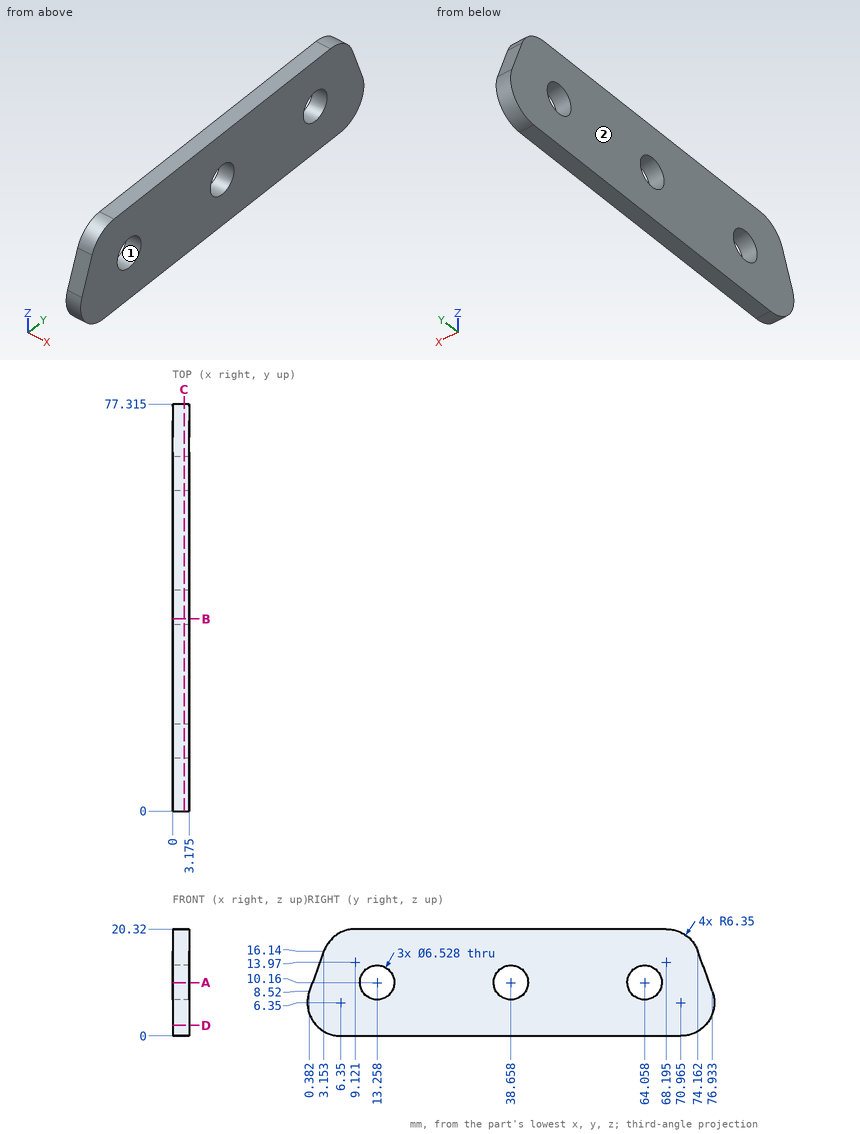
Check sheet for the drawn part. Datum: minimum x, y, z corner. Units: mm. Round coordinates to 2 decimals unless told otherwise and drop trailing zeros. Order: outer loops, then holes, each group sorted by start corner. A loop starts at its lowest first (then second) coordinate and runs counter-clockwise, first axis right, second up. Notation, with made-up numbers: (-11, 16.25) -> (28, 16.25) arc R19 cw to (28, 42.25) -> close; hole circle Ø8 at (12.25, -12). An arc over 180 degrees is marked (long way). Put each result on its own line as item: value.
1) Section check D-D (z = 2). Record the cut outline in (x, y) (1 decimal).
Final values:
outline: (0, 1.7) -> (3.2, 1.7) -> (3.2, 75.6) -> (0, 75.6) -> close
2) Mould release check, pull along Y, two halves, no side actions. Record for the marked faces 1 and 2: +Y half, -Y half, draft (parallel to the pull), parting line (faces both ways), or undercut.
Final values:
face 1: undercut
face 2: draft
3) Material ranges on line 1 (Y direction, x = 0.7, z = 10.16) (1 decimal); line 2 (Z direction, x = 0.55, y = 64); line 3 (Y direction, x = 0.55, z = 6.75), recorded low to high.
Final values:
line 1: y = 1 to 10, 16.5 to 35.4, 41.9 to 60.8, 67.3 to 76.3
line 2: z = 0 to 6.9, 13.42 to 20.32
line 3: y = 0.01 to 77.3
4) Section check B-B (y = 36.5). Record the cut outline in (x, z) (1 decimal).
Final values:
outline: (0, 0) -> (3.2, 0) -> (3.2, 7.7) -> (0, 7.7) -> close; (0, 12.6) -> (3.2, 12.6) -> (3.2, 20.3) -> (0, 20.3) -> close
5) Section check A-A (z = 10.16). Record the cut outline in (x, y) (1 decimal), then the cut area to 3 significant figures.
Final values:
outline: (0, 1) -> (3.2, 1) -> (3.2, 10) -> (0, 10) -> close; (0, 16.5) -> (3.2, 16.5) -> (3.2, 35.4) -> (0, 35.4) -> close; (0, 41.9) -> (3.2, 41.9) -> (3.2, 60.8) -> (0, 60.8) -> close; (0, 67.3) -> (3.2, 67.3) -> (3.2, 76.3) -> (0, 76.3) -> close
area: 177 mm^2
6) Section check C-C (x = 2.2). Give the number of separate pieces and of enclosed holes in the cut face, then the cut area to 3 significant figures.
Final values:
separate pieces: 1
enclosed holes: 3
area: 1,390 mm^2
7) Depth check by flat-ended pin: pin 1 (1.5 mm diameter, centred on x = 2.5, z = 2.5, fed in from -Y). Enter the tip coordinate at first touch or a pass-through.
Final values:
pin 1: stops at y = 0.81
